```python
from build123d import *

# Parameters (mm, degrees)
CHAMFER_1_SIZE           = 1.25
CHAMFER_1_SIZE2          = 0.334936491
SKETCH_2_R               = 2
CUT_EXTRUDE_3_DEPTH      = 1
CUT_EXTRUDE_3_DEPTH_BACK = 8
CHAMFER_2_SIZE           = 1.25
CHAMFER_2_SIZE2          = 0.334936491


with BuildPart() as part:
    # Эскиз1 → Повернуть2 (revolve)
    with BuildSketch(Plane.XY):
        Polygon((0, 0), (37.5, 0), (37.5, 3.5), (3, 3.5), (3, 7), (0, 7), align=None)
    revolve(axis=Axis((0, 7, 0), (0, -1, 0)))

    # Фаска1
    chamfer_1_edges = [part.edges().sort_by_distance(p)[0] for p in [
        (-37.5, 3.5, 0),
    ]]
    chamfer_1_side = [part.faces().sort_by_distance(p)[0] for p in [
        (-36.439339828, 3.5, 0),
    ]]
    chamfer(chamfer_1_edges, length=CHAMFER_1_SIZE, length2=CHAMFER_1_SIZE2, reference=chamfer_1_side[0])

    # Эскиз2 → Вырез-Вытянуть3 (cut, two sides)
    with BuildSketch(Plane(origin=(0, 0, 0), x_dir=(-1, 0, 0), z_dir=(0, -1, 0))) as cut_extrude_3_sk:
        Circle(SKETCH_2_R)
    extrude(amount=CUT_EXTRUDE_3_DEPTH, mode=Mode.SUBTRACT)
    extrude(cut_extrude_3_sk.sketch, amount=-CUT_EXTRUDE_3_DEPTH_BACK, mode=Mode.SUBTRACT)

    # Фаска2
    chamfer_2_edges = [part.edges().sort_by_distance(p)[0] for p in [
        (-37.5, 0, 0),
    ]]
    chamfer_2_side = [part.faces().sort_by_distance(p)[0] for p in [
        (-36.439339828, 0, 0),
    ]]
    chamfer(chamfer_2_edges, length=CHAMFER_2_SIZE, length2=CHAMFER_2_SIZE2, reference=chamfer_2_side[0])


solid = part.part
```
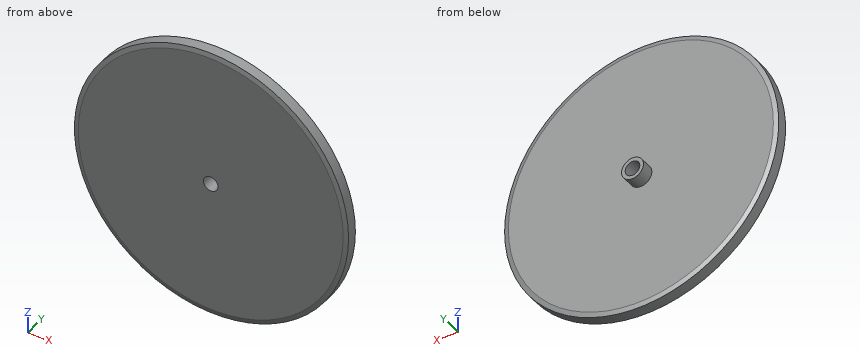
Work out the finished part from the listing and answer in its coordinate system (mm). Round coordinates to 2 decimals unless told otherwise and drop trailing zeros. Write each loop counter-clockwise with the first axis right and the second up, starting at its lowest first coordinate (ties: lowest second). Pieces come first, ordered by that corner, then holes.
1) Consider probe 1 along Z at (x, y) = (0, 3); probe 2 along Y at (x, z) = (22.5, 25); probe 3 along X at (y, z) = (4.5, -0.5). Determine where each line is inside the solid, lowest interval first.
2) Flat-ended cylindrical pins translate along their axes: P1, Ø2, axis at x = -17, z = -23, coming from the -Y side; P2, Ø2, axis at y = 2.5, z = -25.5, coming from the -X side. Find the tip coordinate at first contact, or state that the pin passes through.
3) A cutting plane is placed at B-B on z = 0. Determine the outline of the cut face in (x, y), and give its area (3 significant figures).
4) A cutting plane is placed at A-A on x = 0. Determine the outline of the cut face in (y, z).
5) A cutting plane is placed at C-C on y = 4.5. Determine the outline of the cut face in (x, z), and give its area (3 significant figures).
Entries:
1. probe 1: z = -37.5 to -2, 2 to 37.5
1. probe 2: y = 0 to 3.5
1. probe 3: x = -2.96 to -1.94, 1.94 to 2.96
2. P1: stops at y = 0
2. P2: stops at x = -28.39
3. outline: (-37.5, 0.33) - (-36.25, 0) - (-2, 0) - (-2, 7) - (-3, 7) - (-3, 3.5) - (-36.25, 3.5) - (-37.5, 3.17) - close; (2, 0) - (36.25, 0) - (37.5, 0.33) - (37.5, 3.17) - (36.25, 3.5) - (3, 3.5) - (3, 7) - (2, 7) - close
3. area: 255 mm2
4. outline: (0, -36.25) - (0.33, -37.5) - (3.17, -37.5) - (3.5, -36.25) - (3.5, -3) - (7, -3) - (7, -2) - (0, -2) - close; (0, 2) - (7, 2) - (7, 3) - (3.5, 3) - (3.5, 36.25) - (3.17, 37.5) - (0.33, 37.5) - (0, 36.25) - close
5. outline: circle Ø6 at (0, 0); hole circle Ø4 at (0, 0)
5. area: 15.7 mm2
